from build123d import *

# Parameters (mm, degrees)
SKETCH036_W            = 40
SKETCH036_H            = 40
PAD009_DEPTH           = 11
SKETCH037_W            = 0.75
SKETCH037_H            = 13.12
POCKET009_DEPTH        = 20.001
POCKET009_DEPTH_BACK   = 20.001
LINEARPATTERN002_COUNT = 25
LINEARPATTERN002_PITCH = 1.541667


with BuildPart() as part:
    # Sketch036 → Pad009 (new body)
    with BuildSketch(Plane.XY):
        Rectangle(SKETCH036_W, SKETCH036_H)
    extrude(amount=PAD009_DEPTH)

    # Sketch037 → Pocket009 (cut, two sides)
    with BuildSketch(Plane.XZ) as pocket009_sk:
        with Locations((-18.625, 8.31)):
            Rectangle(SKETCH037_W, SKETCH037_H)
    pocket009 = extrude(amount=-POCKET009_DEPTH, mode=Mode.SUBTRACT) + extrude(pocket009_sk.sketch, amount=POCKET009_DEPTH_BACK, mode=Mode.SUBTRACT)

    # LinearPattern002: Pocket009 ×25
    with Locations(*[(i * LINEARPATTERN002_PITCH, 0, 0) for i in range(1, LINEARPATTERN002_COUNT)]):
        add(pocket009, mode=Mode.SUBTRACT)


with BuildPart() as part_1:
    # Body022 placement: moved
    add(part.part.moved(Location((0, 0, 4))))


solid = part_1.part
Can you work these out from the model? Positions are in its coordinate system, mm. A direction names the side the tool comes from. Give positions to 0.01 mm unless a question says otherwise; leave off trailing zeros. One line per item, written item: value. Start each with the question number.
1) On a 3-axis mill with a long thin cutter (end or side, diameter ignored), from which of +Z, -Z, +X, -X, +Y, -Y can I reach the whole of each face in a straight line? I mean faces 1 (the face through (-1.292, 0, 10)), 2 (the face through (0, 0, 4)). Say none if no direction works.
2) Thinking about a two-plate mould opening in X: for faces 3 (the face through (20, 0, 9)), 4 (the face through (0, -20, 5)), 5 (the face through (-6.667, 0, 10)), 6 (the face through (-13.625, 0, 10)), which applies, +X half, -X half, draft (parallel to the pull), parting line (faces both ways), or undercut?
3) If we section it at A-A, the plane z = 13.75: Give the number of separate pieces and of enclosed holes in the cut face, and give its area (3 significant figures).
4) If I drill on line 1 (Z direction, x = -4.5, y = -6.5), over which ranges is the centre line in solid material (lowest first)? Write a range as [from, to].
Completed:
1. face 1: +Z, +Y, -Y
1. face 2: -Z, +X, -X, +Y, -Y
2. face 3: +X half
2. face 4: draft
2. face 5: undercut
2. face 6: undercut
3. separate pieces: 26
3. enclosed holes: 0
3. area: 850 mm^2
4. line 1: z = [4, 5.75]
